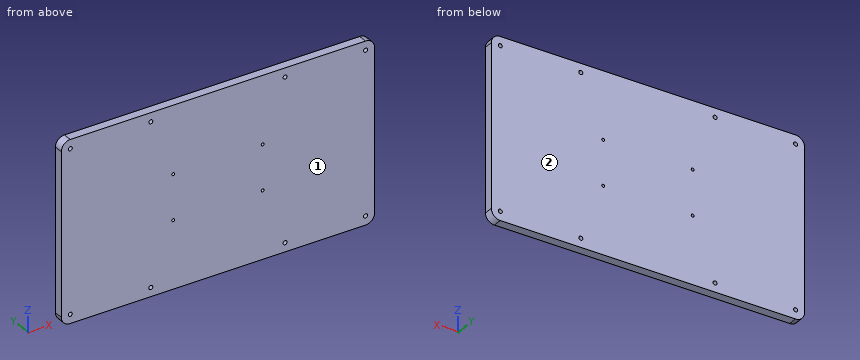
from build123d import *

# Parameters (mm, degrees)
SKETCH_1_W        = 350
SKETCH_1_H        = 200
EXTRUDE_1_DEPTH   = 10
M4X0_7_D          = 3.3
HOLE_WIZARD_M42_D = 4.5
FILLET_1_R        = 10


with BuildPart() as part:
    # Эскиз1 → Бобышка-Вытянуть1 (new body)
    with BuildSketch(Plane(origin=(0, 0, 0), x_dir=(1, 0, 0), z_dir=(0, 1, 0))):
        with Locations((175, 100)):
            Rectangle(SKETCH_1_W, SKETCH_1_H)
    extrude(amount=EXTRUDE_1_DEPTH)

    # Отверстие обработанное метчиком M4x0.7 (through all)
    with Locations(Plane(origin=(134.244811271, 10, -121.125670736), x_dir=(0, 0, -1), z_dir=(0, 1, 0))):
        with Locations((-46.125670736, 9.244811271), (3.874329264, 9.244811271), (3.874329264, -90.755188729), (-46.125670736, -90.755188729)):
            Hole(M4X0_7_D / 2)

    # Отверстие с зазором M42 (through all)
    with Locations(Plane(origin=(0, 10, 0), x_dir=(1, 0, 0), z_dir=(0, 1, 0))):
        with Locations((10, 10), (100, 10), (100, 190), (10, 190), (250, 190), (340, 190), (340, 10), (250, 10)):
            Hole(HOLE_WIZARD_M42_D / 2)

    # Скругление1
    fillet_1_edges = [part.edges().sort_by_distance(p)[0] for p in [
        (0, 5, -200),
        (350, 5, -200),
        (350, 5, 0),
        (0, 5, 0),
    ]]
    fillet(fillet_1_edges, radius=FILLET_1_R)


solid = part.part
Check sheet for the modelled part. Datum: model origin and axes. Units: mm. Face numbers are marked on the shaded views. Round coordinates to 2 decimals unless told otherwise and drop trailing zeros.
Q1. Draft check along Y on the marked faces 1 and 2. Enter one of: pulls with the +Y half, pulls with the -Y half, needs draft (parallel to the pull), parting line crosses it, or undercut.
Filled sheet:
face 1: pulls with the -Y half
face 2: pulls with the +Y half
Q2. Scan lines: L1, parallel to X at y = 4, z = -190; L2, parallel to Z at x = 225, y = 2.25; L3, parallel to Z at x = 10, y = 2.75. Record each from-to range of solid material in increasing order.
Filled sheet:
L1: x = 0 to 7.75, 12.25 to 97.75, 102.25 to 247.75, 252.25 to 337.75, 342.25 to 350
L2: z = -200 to -126.65, -123.35 to -76.65, -73.35 to 0
L3: z = -200 to -192.25, -187.75 to -12.25, -7.75 to 0
Q3. Depth check by flat-ended pin: P1, Ø4, axis at x = 225, z = -75, coming from the -Y side; P2, Ø2, axis at x = 125, z = -125, coming from the -Y side. Enter the tip coordinate at first touch or a pass-through.
Filled sheet:
P1: stops at y = 0
P2: passes through
